The model under review builds one solid part; all positions refer to its coordinate system, in mm. A direction names the side the tool comes from. Give positions to 0.01 mm unless a question says otherwise; leave off trailing zeros. Order: outer loops, then holes, each group sorted by start corner. A loop starts at its lowest first (then second) coordinate and runs counter-clockwise, first axis right, second up. Notation, with made-up numbers: M 46.5,8 L 105.5,8 A26 cw 105.5,41 Z; hole C -12,64.25 d1. An arc over 180 degrees is marked long. One line per question, with ' | ' between items. Start each with the question number.
1. We need section D-D on x = 4.5. Write out the cut boundary in (y, z), then the cut area to 3 significant figures.
2. For faces 4 (the face through (7.6, 3.1, 5.8)), 5 (the face through (-11.76, 4.63, 3.3)), list the 3-axis set-ups (+Z, -Z, +X, -X, +Y, -Y) from which the entire face can be reached by the end or side of a thin tool; tool diameter is ignored.
3. We need section B-B on z = 3. Write out the cut boundary in (x, y), then the cut area to 3 significant figures.
4. We need section A-A on y = -12. Write out the cut boundary in (x, z).
5. We need section C-C on x = -8.5. Write out the cut boundary in (y, z), then the cut area to 3 significant figures.
6. The part is to be moulded in two halves that separate along Y. For faces 1 (the face through (1.6, 3.1, 5.8)), 2 (the face through (0, 0, 0)), 3 (the face through (-7.5, 10, 3.2)), say which applies: +Y half, -Y half, draft (parallel to the pull), parting line (faces both ways), or undercut.
7. Insertion check: P1, Ø0.8, axis at y = 2, z = 6, coming from the -X side; P2, Ø0.8, axis at y = 3.5, z = 6.5, coming from the -X side; P3, Ø0.7, axis at x = -12, z = 6, coming from the +Y side. Each pin has a flat end and moves straight along its axis. Give the tip position at first contact, or say it passes through.
8. Wall thickness on L1, parallel to Y at x = 4.5, z = 1.5; L2, parallel to Z at x = -6, y = 3; L3, parallel to X at y = 1, z = 0.75: over which ranges is each line inside the solid? List them lowest first.
```python
from build123d import *

# Parameters (mm, degrees)
F0_W        = 25
F0_H        = 30
F1_DEPTH    = 6.5
F2_R        = 1.5
F3_DEPTH    = 6.501
F4_W        = 1
F4_H        = 6.1
F4_W_2      = 0.4
F4_W_3      = 0.6
F5_DEPTH    = 0.7
F6_T1_DEPTH = 57.9336597593
F7_R        = 10


# Not quite as in the source:
# - a fillet or chamfer that OpenCascade refuses, or shapes differently, is made with other operations: its cross-section is extruded or revolved along the edge and cut away or added


with BuildPart() as f1:
    # F0 (on Top) → F1 (new body)
    with BuildSketch(Plane.XY):
        Rectangle(F0_W, F0_H)
    extrude(amount=F1_DEPTH)

    # F2 (on face) → F3 (cut, through all)
    with BuildSketch(Plane.XY.offset(6.5)):
        with Locations((-2, -12)):
            Circle(F2_R)
        with Locations((4.5, -1.5)):
            Circle(F2_R)
        with Locations((4.5, 8.5)):
            Circle(F2_R)
    extrude(amount=-F3_DEPTH, mode=Mode.SUBTRACT)

    # F4 (on face) → F5 (cut)
    with BuildSketch(Plane.XY.offset(6.5)):
        with Locations((11.6, 3.051)):
            Rectangle(F4_W, F4_H)
        with Locations((9.6, 3.051)):
            Rectangle(F4_W, F4_H)
        with Locations((7.6, 3.051)):
            Rectangle(F4_W, F4_H)
        with Locations((5.6, 3.051)):
            Rectangle(F4_W, F4_H)
        with Locations((3.6, 3.051)):
            Rectangle(F4_W, F4_H)
        with Locations((1.6, 3.051)):
            Rectangle(F4_W, F4_H)
        with Locations((-0.4, 3.051)):
            Rectangle(F4_W, F4_H)
        with Locations((-2.4, 3.051)):
            Rectangle(F4_W, F4_H)
        with Locations((-4.4, 3.051)):
            Rectangle(F4_W, F4_H)
        with Locations((-6.4, 3.051)):
            Rectangle(F4_W, F4_H)
        with Locations((-8.4, 3.051)):
            Rectangle(F4_W, F4_H)
        with Locations((-10.4, 3.051)):
            Rectangle(F4_W, F4_H)
        with Locations((-12.7, 3.051)):
            Rectangle(F4_W_2, F4_H)
        with Locations((-12.2, 3.051)):
            Rectangle(F4_W_3, F4_H)
    extrude(amount=-F5_DEPTH, mode=Mode.SUBTRACT)

    # F6: chamfer of 10 on 1 edges, made by hand

    # F6_s2 → F6_t1 (cut)
    with BuildSketch(Plane.XY.offset(-25.7168298797)):
        Polygon((-12.5, 5), (-2.5, 15), (-12.5, 15), align=None)
    extrude(amount=F6_T1_DEPTH, mode=Mode.SUBTRACT)

    # F7
    f7_edges = [f1.edges().sort_by_distance(p)[0] for p in [
        (-2.5, 15, 3.25),
        (-12.5, 5, 2.9),
        (12.5, 15, 3.25),
    ]]
    fillet(f7_edges, radius=F7_R)


solid = f1.part
```
Entries:
1) outline: M -15,0 L -3,0 L -3,6.5 L -15,6.5 Z; M 0,0 L 7,0 L 7,6.5 L 0,6.5 Z; M 10,0 L 14.8,0 L 14.8,6.5 L 10,6.5 Z | area: 155 mm^2
2) face 4: +Z | face 5: +Z, -Z, -X, +Y
3) outline: M -12.5,-15 L 12.5,-15 L 12.5,5 A10 ccw 2.5,15 L 1.64,15 A10 ccw -5.43,12.07 L -9.57,7.93 A10 ccw -12.5,0.86 Z; hole C -2,-12 d3; hole C 4.5,-1.5 d3; hole C 4.5,8.5 d3 | area: 653 mm^2
4) outline: M -12.5,0 L -3.5,0 L -3.5,6.5 L -12.5,6.5 Z; M -0.5,0 L 12.5,0 L 12.5,6.5 L -0.5,6.5 Z
5) outline: M -15,0 L 9,0 L 9,6.5 L 6.1,6.5 L 6.1,5.8 L 0,5.8 L 0,6.5 L -15,6.5 Z | area: 152 mm^2
6) face 1: undercut | face 2: draft | face 3: +Y half
7) P1: stops at x = -12.47 | P2: stops at x = -11.9 | P3: stops at y = 4.89
8) L1: y = -15 to -3, 0 to 7, 10 to 14.8 | L2: z = 0 to 5.8 | L3: x = -12.5 to 12.5
